Study the drawing (mm; zero at the part's minimum x, y, z) and answer. A direction names the side the tool comes from. Coordinates: 2 decimals unless noted, no trailing zeros. Write each loop counter-clockwise with the first axis right and the second up, starting at its lowest first coordinate (ties: lowest second). Pieces come first, ordered by that corner, then holes. Notation, with made-up numbers: M 65,-15.75 L 112,-15.75 A6 cw 112,-8.75 Z; hole C 22.25,25 d11. An arc over 180 degrees is marked long. Answer as a JSON object with one key per item and string values. Group by question number.
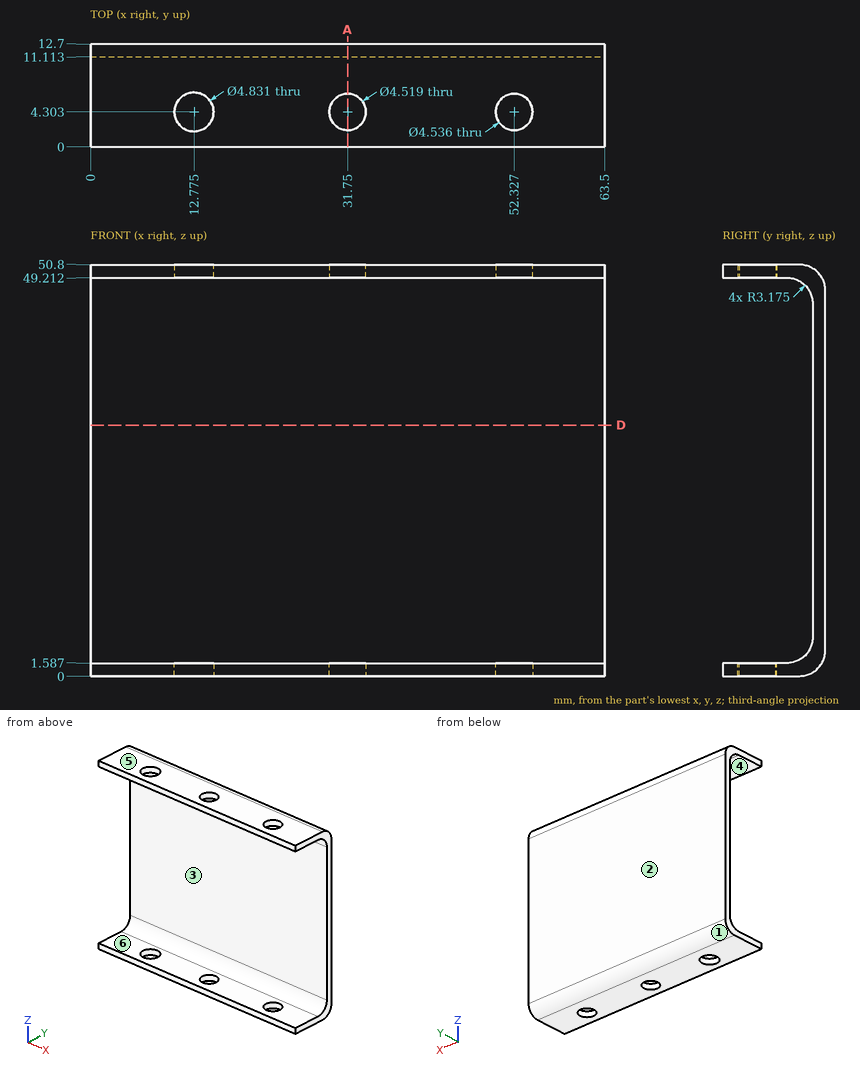
Item 1: A cutting plane is placed at D-D, the plane z = 31. Write down the section's boundary in (x, y).
Item 2: Consider L1, parallel to Z at x = 10, y = 4; L2, parallel to Y at x = 30, z = 38.5; L3, parallel to Y at x = 27, z = 2.5 (1 decimal). Determine where each line is inside the solid, lowest interval first. Write a range as from..to.
Item 3: A cutting plane is placed at A-A, the plane x = 31.75. State how many separate pieces and enclosed holes the cut face has.
Item 4: A tool of negligible diameter and unlimited length cuts with its end or side. For the marked faces 5 and 6, from which of +Z, -Z, +X, -X, +Y, -Y can it reach the whole face along a straight path? Write none if from no direction.
Item 5: For a pull along Z with two mould halves and no side action, classify the marked faces 1, 2, 3 and 4 as +Z half, -Z half, draft (parallel to the pull), parting line (faces both ways), or undercut.
Item 6: Flat-ended cylindrical pins translate along their axes: pin 1 Ø2 at (x, z) = (15, 42) entering from -Y; pin 2 Ø1 at (x, y) = (22, 8.5) entering from -Z; pin 3 Ø2.5 at (x, y) = (52.33, 4.3) entering from +Z. Find the tip coordinate at first contact, or state that the pin passes through.
Answer:
{
 "1": {"outline": "M 0,11.11 L 63.5,11.11 L 63.5,12.7 L 0,12.7 Z"},
 "2": {"L1": "0..1.59, 49.21..50.8", "L2": "11.11..12.7", "L3": "10.2..12.6"},
 "3": {"separate pieces": "3", "enclosed holes": "0"},
 "4": {"face 5": "+Z, +X, -X, +Y, -Y", "face 6": "+X, -X, -Y"},
 "5": {"face 1": "-Z half", "face 2": "draft", "face 3": "undercut", "face 4": "undercut"},
 "6": {"pin 1": "y = 11.11", "pin 2": "z = 0", "pin 3": "through"}
}
